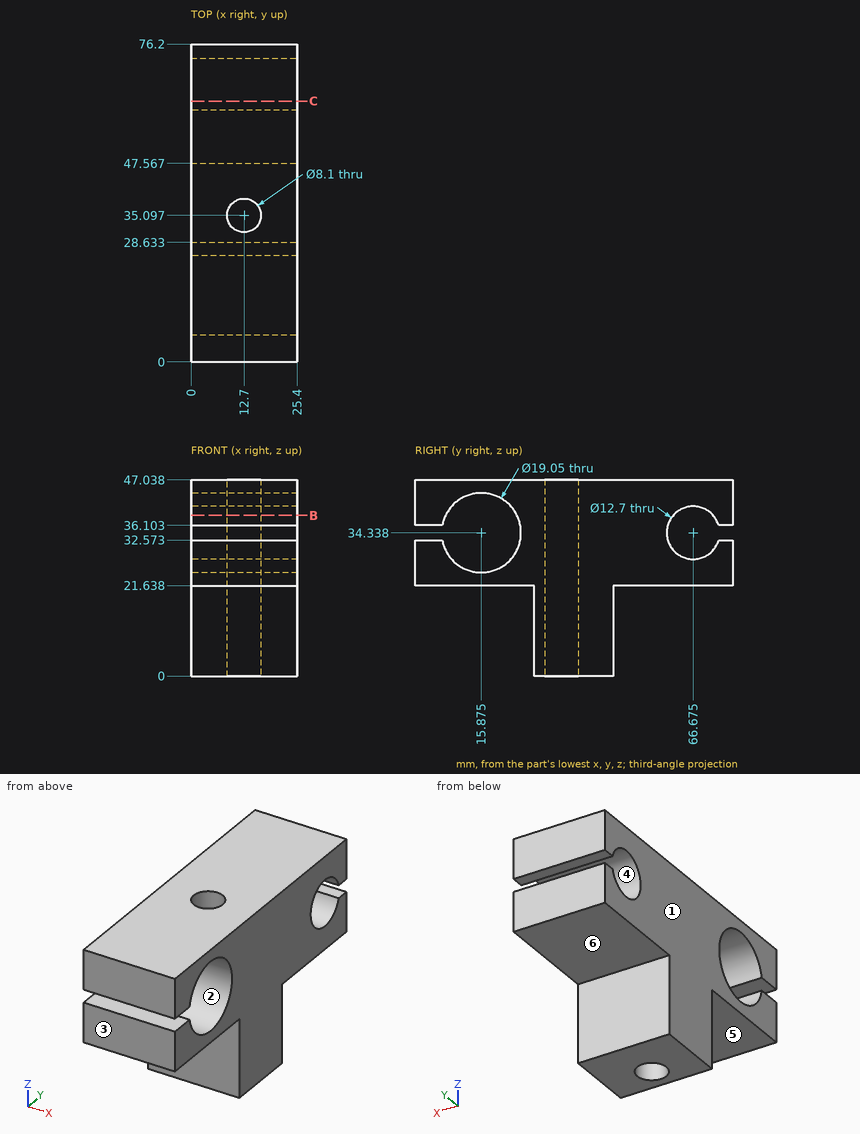
Source: three-view drawing plus pictorial views. Frame: mm from the lowest corner of the part. A direction names the side the tool comes from. Give positions to 0.01 mm unless a question says otherwise; leave off trailing zeros. Write each loop counter-clockwise with the first axis right and the second up, starting at its lowest first coordinate (ties: lowest second). Pieces come first, ordered by that corner, then holes.
(1) Cut plane C-C, the plane y = 62.5. Return loops of the section in (x, z).
(2) Mould query, pull axis Y, two halves, no side actions, for the marked faces 1, 2 and 3. Classes: released by +Y, released by -Y, zero draft, split by the parting line, or undercut.
(3) Cut plane B-B, the plane z = 38.5. Return loops of the section in (x, y).
(4) Ray query, line 1 (Z direction, x = 2.75, y = 15.5) (1 decimal); line 2 (Y direction, x = 12.75, z = 15); line 3 (Y direction, x = 2.25, z = 12). Return the intervals inside material, ascending.
(5) Access query for the marked faces 4, 5 and 6. Directions: +Z, -Z, +X, -X, +Y, -Y. A direction counts if a zero-diameter tool reaches every point of the face in a straight line with its end or side. Return the directions, or none.
(6) First-contact query: P1, Ø8, axis at x = 15.5, z = 9, coming from the +Y side; P2, Ø10, axis at x = 22.5, z = 9, coming from the -Y side; P3, Ø1, axis at x = 13.5, y = 56, coming from the -Z side. Flat tips, straight axial feed; report the tip coordinate or a pass-through.
Values follow:
1. outline: (0, 21.64) - (25.4, 21.64) - (25.4, 29.55) - (0, 29.55) - close; (0, 39.12) - (25.4, 39.12) - (25.4, 47.04) - (0, 47.04) - close
2. face 1: zero draft
2. face 2: undercut
2. face 3: released by -Y
3. outline: (0, 0) - (25.4, 0) - (25.4, 7.31) - (0, 7.31) - close; (0, 24.44) - (25.4, 24.44) - (25.4, 61.88) - (0, 61.88) - close; (0, 71.47) - (25.4, 71.47) - (25.4, 76.2) - (0, 76.2) - close; hole circle Ø8.1 at (12.7, 35.1)
4. line 1: z = 21.6 to 24.8, 43.9 to 47
4. line 2: y = 28.63 to 31.05, 39.15 to 47.57
4. line 3: y = 28.63 to 47.57
5. face 4: +X, -X
5. face 5: -Z, +X, -X, -Y
5. face 6: -Z, +X, -X, +Y
6. P1: stops at y = 47.57
6. P2: stops at y = 28.63
6. P3: stops at z = 21.64
